Could you check a few things on this drawing? It's one solid part, dimensions in mm from its lowest x, y, z. A direction names the side the tool comes from. Give positions to 0.01 mm unless a question says otherwise; leave off trailing zeros. Loops run counter-clockwise (first coordinate to the right, second up) from the corner with the lowest first, then second, coordinate; pieces in that order, holes last. Notation, with made-up numbers: (51, 45.25) - (70, 45.25) arc R7 cw to (70, 55.25) - close; hole circle Ø6 at (72, 36.5). An arc over 180 degrees is marked (long way). Write each question's results on one line, items separated by ' | '. Start each with the question number.
(1) Suppose I cut it at D-D (z = 60). Please give me the cut outline in (x, y).
(2) On a 3-axis mill with a long thin cutter (end or side, diameter ignored), from which of +Z, -Z, +X, -X, +Y, -Y can I reach the whole of each face in a straight line? I mean the marked faces 1, 2, 3 and 4. Say none if no direction works.
(3) Suppose I cut it at B-B (x = 19). Please give me the cut outline in (y, z), and give its area (3 significant figures).
(4) Suppose I cut it at C-C (y = 9.5). Please give me the cut outline in (x, z).
(5) For pin 1 (17 mm diameter, centred on x = 17, z = 27, fed in from -Y); pin 2 (4.5 mm diameter, centred on x = 3.5, y = 18, fed in from +Z); pin 3 (7 mm diameter, centred on y = 21.5, z = 38, fed in from +X), each with a flat end and sliding along its axis, tell me the tip position at first contact or that it passes through.
(6) I need wall thicknesses on line 1 (X direction, y = 23.75, z = 40.5); line 2 (X direction, y = 3, z = 13.5); line 3 (Y direction, x = 24, z = 25). Which ranges of each line are inside material? Lowest first, please.
(7) If we mould it in two halves opening along X, with no side actions, what happens to the marked faces 5, 6 and 7? For each: released by +X, released by -X, zero draft, split by the parting line, or undercut.
(8) Suppose I cut it at A-A (z = 37). Please give me the cut outline in (x, y), and give its area (3 significant figures).
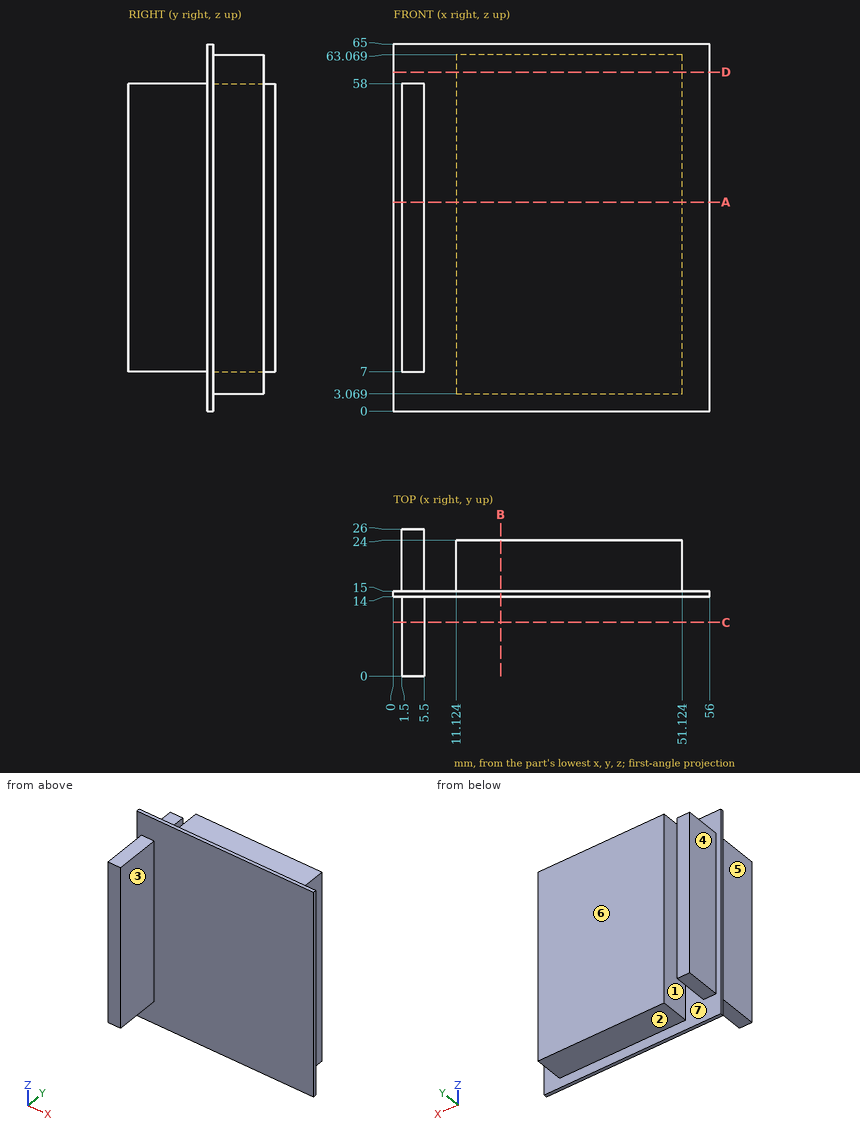
Output values:
1) outline: (0, 14) - (56, 14) - (56, 15) - (51.12, 15) - (51.12, 24) - (11.12, 24) - (11.12, 15) - (0, 15) - close
2) face 1: +Z, -Z, +Y | face 2: -Z, +X, -X, +Y | face 3: +Z, -Z, +X, -Y | face 4: +Z, -Z, -X, +Y
3) outline: (14, 0) - (15, 0) - (15, 3.07) - (24, 3.07) - (24, 63.07) - (15, 63.07) - (15, 65) - (14, 65) - close | area: 605 mm2
4) outline: (1.5, 7) - (5.5, 7) - (5.5, 58) - (1.5, 58) - close
5) pin 1: y = 14 | pin 2: z = 58 | pin 3: x = 51.12
6) line 1: 1.5 to 5.5, 11.12 to 51.12 | line 2: 1.5 to 5.5 | line 3: 14 to 24
7) face 5: released by -X | face 6: zero draft | face 7: undercut
8) outline: (0, 14) - (1.5, 14) - (1.5, 0) - (5.5, 0) - (5.5, 14) - (56, 14) - (56, 15) - (51.12, 15) - (51.12, 24) - (11.12, 24) - (11.12, 15) - (5.5, 15) - (5.5, 26) - (1.5, 26) - (1.5, 15) - (0, 15) - close | area: 516 mm2
